Source: CAD feature listing. Evaluate the final solid. Frame: model axes, mm. A direction names the side the tool comes from. Give positions to 0.01 mm unless a question says otherwise; leave off trailing zeros. Loops run counter-clockwise (first coordinate to the right, second up) from the corner with the lowest first, then second, coordinate; pieces in that order, holes last. Notation, with made-up numbers: M -3,35 L 54,35 A21 ccw 54,45 Z; hole C 3.25,-39 d10. An arc over 180 degrees is marked long. Answer in a Markdown table with one row per item.
```python
from build123d import *

# Parameters (mm, degrees)
F1_DEPTH = 12
F2_R     = 3
F3_DEPTH = 12.001
F4_R     = 0.75
F5_DEPTH = 5
F6_R     = 2.5
F7_DEPTH = 12.001


with BuildPart() as f1:
    # F0 (on Front) → F1 (new body)
    with BuildSketch(Plane.XZ):
        Polygon((9.200479, 21.225578), (-35.799521, 21.225578), (-35.799521, 9.225578), (39.200479, 9.225578), (39.200479, 11.725578), align=None)
    extrude(amount=-F1_DEPTH)

    # F2 (on face) → F3 (cut, through all)
    with BuildSketch(Plane.XY.offset(21.225578)):
        with Locations((0, 6)):
            Circle(F2_R)
    extrude(amount=-F3_DEPTH, mode=Mode.SUBTRACT)

    # F4 (on face) → F5 (cut)
    with BuildSketch(Plane.XY.offset(21.225578)):
        with Locations((-5.799521, 6)):
            Circle(F4_R)
    extrude(amount=-F5_DEPTH, mode=Mode.SUBTRACT)

    # F6 (on face) → F7 (cut, through all)
    with BuildSketch(Plane(origin=(0, 0, 9.225578), x_dir=(1, 0, 0), z_dir=(0, 0, -1))):
        with Locations((-27.799521, -6)):
            Circle(F6_R)
    extrude(amount=-F7_DEPTH, mode=Mode.SUBTRACT)


solid = f1.part
```
Q1. Section query D-D (z = 20.25). Output: boundary loops of the cut face in (x, y).
Values follow:
| item | result |
|---|---|
| outline | M -35.8,0 L 12.28,0 L 12.28,12 L -35.8,12 Z; hole C -27.8,6 d5; hole C -5.8,6 d1.5; hole C 0,6 d6 |
Q2. Reachability of faces 1 (the cylindrical face through (-25.49, 6.96, 15.14)), 2 (the flat face through (-6, 6, 16.226)) from +Z, -Z, +X, -X, +Y, -Y: full face, straight path, thin tool, end or side. Return the list, or none.
Values follow:
| item | result |
|---|---|
| face 1 | +Z, -Z |
| face 2 | +Z |
Q3. Contact query for a flat-ended pin moving along its axis: pin 1 Ø3 at (x, y) = (30, 6) entering from +Z. Output: stop coordinate, or through.
Values follow:
| item | result |
|---|---|
| pin 1 | z = 15.11 |
Q4. Section query C-C (z = 10.5). Output: boundary loops of the cut face in (x, y), plus the area to 3 significant figures.
Values follow:
| item | result |
|---|---|
| outline | M -35.8,0 L 39.2,0 L 39.2,12 L -35.8,12 Z; hole C -27.8,6 d5; hole C 0,6 d6 |
| area | 852 mm^2 |
Q5. Section query B-B (y = 6). Output: boundary loops of the cut face in (x, z).
Values follow:
| item | result |
|---|---|
| outline | M -35.8,9.23 L -30.3,9.23 L -30.3,21.23 L -35.8,21.23 Z; M -25.3,9.23 L -3,9.23 L -3,21.23 L -5.05,21.23 L -5.05,16.23 L -6.55,16.23 L -6.55,21.23 L -25.3,21.23 Z; M 3,9.23 L 39.2,9.23 L 39.2,11.73 L 9.2,21.23 L 3,21.23 Z |
Q6. Ray query, probe 1 along Y at (x, z) = (0, 18); probe 2 along X at (y, z) = (5, 11.5); probe 3 along Z at (x, y) = (25, 3). Return the intervals inside material, ascending. Write a range as from..to.
Values follow:
| item | result |
|---|---|
| probe 1 | 0..3, 9..12 |
| probe 2 | -35.8..-30.09, -25.51..-2.83, 2.83..39.2 |
| probe 3 | 9.23..16.22 |
Q7. Mould query, pull axis X, two halves, no side actions, for faces 3 (the flat face through (1, 2, 9.226)), 4 (the flat face through (-35.8, 6, 15)), 5 (the cylindrical face through (-0.65, 3.07, 15.31)), 6 (the flat face through (24.41, 5.92, 16.41)). Classes: +X half, -X half, draft (parallel to the pull), parting line (faces both ways), or undercut.
Values follow:
| item | result |
|---|---|
| face 3 | draft |
| face 4 | -X half |
| face 5 | undercut |
| face 6 | +X half |
Q8. Section query A-A (x = 0). Output: boundary loops of the cut face in (y, z).
Values follow:
| item | result |
|---|---|
| outline | M 0,9.23 L 3,9.23 L 3,21.23 L 0,21.23 Z; M 9,9.23 L 12,9.23 L 12,21.23 L 9,21.23 Z |
